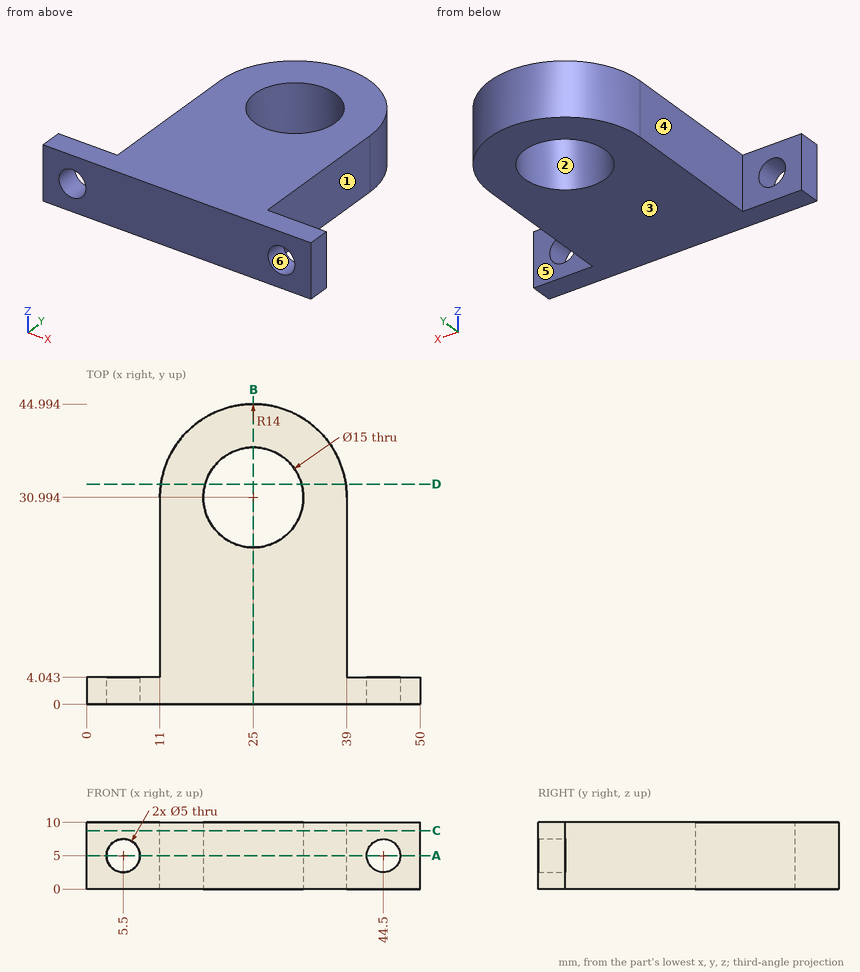
Study the drawing (mm; zero at the part's minimum x, y, z) and answer. A direction names the side the tool comes from. Give positions to 0.01 mm unless a question says otherwise; leave off trailing zeros. Loops run counter-clockwise (first coordinate to the right, second up) from the corner with the lowest first, then second, coordinate; pieces in that order, holes last. Notation, with made-up numbers: M 74.5,3.5 L 129.5,3.5 A26 cw 129.5,27.5 Z; hole C -6,29 d2. An arc over 180 degrees is marked long. Use CSV: the item, a comma, the result in double quotes.
1) Which of the six approach directions +Z, -Z, +X, -X, +Y, -Y give full straight-line access (tool end or side, diameter ignored) to the marked faces 4, 5 and 6?
Answer:
face 4,"+Z, -Z, -X, +Y"
face 5,"+Z, -Z, +X, +Y"
face 6,"+Y, -Y"
2) Determine the mould class of the marked faces 1, 2 and 3 for opening direction X: released by +X, released by -X, zero draft, split by the parting line, or undercut.
Answer:
face 1,"released by +X"
face 2,"undercut"
face 3,"zero draft"
3) Find section C-C on z = 8.75. Write down the section's boundary in (x, y), plus the area to 3 significant figures.
Answer:
outline,"M 0,0 L 50,0 L 50,4.04 L 39,4.04 L 39,30.99 A14 ccw 11,30.99 L 11,4.04 L 0,4.04 Z; hole C 25,30.99 d15"
area,"1,090 mm^2"
4) Find section D-D on y = 33. Write down the section's boundary in (x, z) (1 decimal).
Answer:
outline,"M 11.1,0 L 17.8,0 L 17.8,10 L 11.1,10 Z; M 32.2,0 L 38.9,0 L 38.9,10 L 32.2,10 Z"
5) Find section A-A on z = 5. Write down the section's boundary in (x, y), plus the area to 3 significant figures.
Answer:
outline,"M 0,0 L 3,0 L 3,4.04 L 0,4.04 Z; M 8,0 L 42,0 L 42,4.04 L 39,4.04 L 39,30.99 A14 ccw 11,30.99 L 11,4.04 L 8,4.04 Z; M 47,0 L 50,0 L 50,4.04 L 47,4.04 Z; hole C 25,30.99 d15"
area,"1,050 mm^2"
6) Find section B-B on x = 25. Write down the section's boundary in (y, z).
Answer:
outline,"M 0,0 L 23.49,0 L 23.49,10 L 0,10 Z; M 38.49,0 L 44.99,0 L 44.99,10 L 38.49,10 Z"
7) Consider L1, parallel to Y at x = 25, z = 4.5; L2, parallel to Z at x = 5.5, y = 1.7; L3, parallel to X at y = 6.5, z = 2.75. Determine where each line is inside the solid, lowest interval first.
Answer:
L1,"0 to 23.49, 38.49 to 44.99"
L2,"0 to 2.5, 7.5 to 10"
L3,"11 to 39"
8) Given P1, Ø5, axis at x = 7, z = 5.5, coming from the +Y side; P2, Ø1.5, axis at y = 33.5, z = 3, coming from the +X side; P3, Ø6, axis at y = 21.5, z = 2.5, coming from the +X side, each flat-ended and moving along its own axis, determine where each tip first touches the part or whether it passes through.
Answer:
P1,"y = 4.04"
P2,"x = 38.89"
P3,"x = 39"
